Source: three-view drawing plus pictorial views. Frame: mm from the lowest corner of the part. Give positions to 0.01 mm unless a question says otherwise; leave off trailing zeros. Order: outer loops, then holes, each group sorted by start corner. A loop starts at its lowest first (then second) coordinate and runs counter-clockwise, first axis right, second up.
1) Draft query along Z for the marked faces 1, 2 and 3. Return one class per face: released by +Z, released by -Z, zero draft, split by the parting line, or undercut.
2) Section A-A, the plane x = 10. Return loops of the section in (y, z) (3 decimals), plus the area to 3 significant figures.
3) Material intervals for line 1 (Z direction, x = 10, y = 8) (3 decimals); line 2 (X direction, y = 8, z = 37.5) (3 decimals); line 3 (X direction, y = 4.5, z = 40), sorted ascending.
4) Section B-B, the plane y = 4.75. Return loops of the section in (x, z) (3 decimals), plus the area to 3 significant figures.
5) First-contact query: P1, Ø8, axis at x = 10, z = 12.5, coming from the -Y side. Flat tip, straight axial feed; report the tip coordinate or a pass-through.
6) Section C-C, the plane z = 12.5. Return loops of the section in (x, y) (3 decimals).
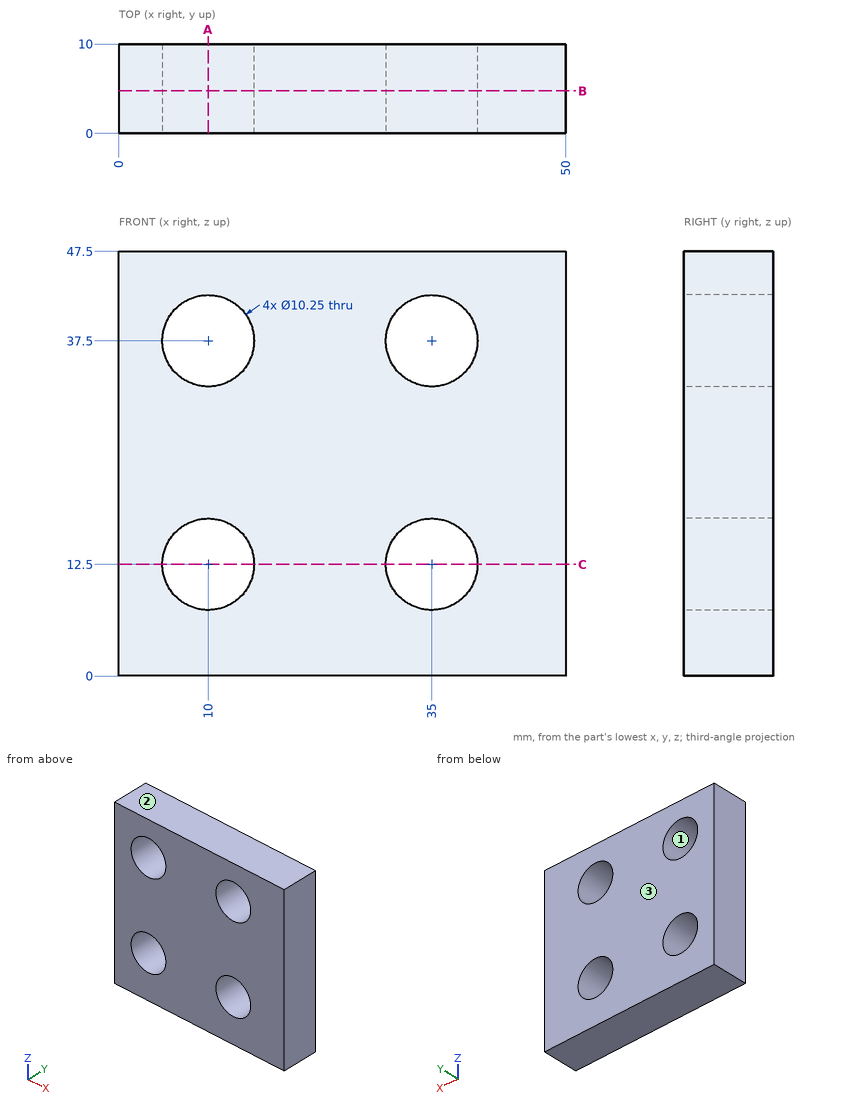
From the geometry:
1. face 1: undercut
1. face 2: released by +Z
1. face 3: zero draft
2. outline: (0, 0) - (10, 0) - (10, 7.375) - (0, 7.375) - close; (0, 17.625) - (10, 17.625) - (10, 32.375) - (0, 32.375) - close; (0, 42.625) - (10, 42.625) - (10, 47.5) - (0, 47.5) - close
2. area: 270 mm2
3. line 1: z = 0 to 7.375, 17.625 to 32.375, 42.625 to 47.5
3. line 2: x = 0 to 4.875, 15.125 to 29.875, 40.125 to 50
3. line 3: x = 0 to 5.53, 14.47 to 30.53, 39.47 to 50
4. outline: (0, 0) - (50, 0) - (50, 47.5) - (0, 47.5) - close; hole circle Ø10.25 at (10, 12.5); hole circle Ø10.25 at (10, 37.5); hole circle Ø10.25 at (35, 12.5); hole circle Ø10.25 at (35, 37.5)
4. area: 2,040 mm2
5. P1: passes through
6. outline: (0, 0) - (4.875, 0) - (4.875, 10) - (0, 10) - close; (15.125, 0) - (29.875, 0) - (29.875, 10) - (15.125, 10) - close; (40.125, 0) - (50, 0) - (50, 10) - (40.125, 10) - close
